from build123d import *

# Parameters (mm, degrees)
F0_W     = 88.9
F0_H     = 88.9
F0_R     = 6.35
F1_DEPTH = 12.7
F2_DEPTH = 76.2
F3_R     = 5.08


with BuildPart() as f1:
    # F0 (on Front) → F1 (new body)
    with BuildSketch(Plane.XZ):
        with Locations((-9.724989, -10.736793)):
            Rectangle(F0_W, F0_H)
        with Locations((-40.30901, -41.320814)):
            Circle(F0_R, mode=Mode.SUBTRACT)
        with Locations((20.859033, -41.320814)):
            Circle(F0_R, mode=Mode.SUBTRACT)
        with Locations((-40.30901, 19.847229)):
            Circle(F0_R, mode=Mode.SUBTRACT)
        with Locations((-9.724989, -10.736793)):
            Circle(F0_R, mode=Mode.SUBTRACT)
        with Locations((20.859033, 19.847229)):
            Circle(F0_R, mode=Mode.SUBTRACT)
    extrude(amount=-F1_DEPTH)

    # F0 (on Front) → F2 (join)
    with BuildSketch(Plane.XZ):
        with Locations((-40.30901, 19.847229)):
            Circle(F0_R)
        with Locations((20.859033, 19.847229)):
            Circle(F0_R)
        with Locations((-9.724989, -10.736793)):
            Circle(F0_R)
        with Locations((20.859033, -41.320814)):
            Circle(F0_R)
        with Locations((-40.30901, -41.320814)):
            Circle(F0_R)
    extrude(amount=-F2_DEPTH)

    # F3
    f3_edges = [f1.edges().sort_by_distance(p)[0] for p in [
        (34.725011, 6.35, 33.713207),
        (-54.174989, 6.35, 33.713207),
        (-54.174989, 6.35, -55.186793),
        (34.725011, 6.35, -55.186793),
        (14.509033, 12.7, 19.847229),
        (-46.65901, 12.7, 19.847229),
        (-16.074989, 12.7, -10.736793),
        (-46.65901, 12.7, -41.320814),
        (14.509033, 12.7, -41.320814),
    ]]
    fillet(f3_edges, radius=F3_R)


solid = f1.part
Verification items for the finished model (mm, model axes). A direction names the side the tool comes from. Round coordinates to 2 decimals unless told otherwise and drop trailing zeros. Loops run counter-clockwise (first coordinate to the right, second up) from the corner with the lowest first, then second, coordinate; pieces in that order, holes last. Notation, with made-up numbers: (9, 15) - (14, 15) arc R17 ccw to (14, 47) - close; hole circle Ø3 at (31.25, -33.5). An arc over 180 degrees is marked (long way). Answer in a Markdown table with one row per item. Add a question column.
Q1. Tool access check on faces 4 (the face through (-10, 76.2, -11)), 5 (the face through (26.916, 46.581, -39.413)). Record the directions out of +Z, -Z, +X, -X, +Y, -Y that give a thin tool (end or side, any length) a straight path to the whole face; none if there is none.
Q2. Material ranges on line 1 (Y direction, x = 25, z = -12.5); line 2 (Z direction, x = -39, y = 30); line 3 (Z direction, x = 19, y = 18), recorded low to high.
Q3. Gauge pin test, flat ends, axial feed: pin 1 (1 mm diameter, centred on y = 23, z = 20, fed in from +X); pin 2 (8 mm diameter, centred on y = 59.5, z = -34.5, fed in from -X); pin 3 (4 mm diameter, centred on x = -34.5, y = 31.5, fed in from +Z). Record the tip position at first contact, or that the pin passes through.
Q4. Section check A-A on y = 65.5. Enter the section's corners in (x, z), plus the area to 3 significant figures.
Q5. Section check C-C on x = -22.5. Enter the section's corners in (y, z).
Q6. Section check B-B on z = -24. Enter the section's corners in (x, y), plus the area to 3 significant figures.
Q7. Release check for a two-part mould opening along X. For faces 1 (the face through (21, 76.2, 20)), 2 (the face through (-41.136, 46.581, 26.143)), 3 (the face through (33.2, 6.44, 32.26)) record: pulls with the +X half, pulls with the -X half, needs draft (parallel to the pull), parting line crosses it, or undercut.
Found:
| question | item | result |
|---|---|---|
| 1 | face 4 | +Z, -Z, +X, -X, +Y |
| 1 | face 5 | +Y |
| 2 | line 1 | y = 0 to 12.7 |
| 2 | line 2 | z = -47.53 to -35.11, 13.63 to 26.06 |
| 2 | line 3 | z = -47.39 to -35.25, 13.78 to 25.92 |
| 3 | pin 1 | stops at x = 27.21 |
| 3 | pin 2 | stops at x = -46 |
| 3 | pin 3 | stops at z = 24.93 |
| 4 | outline | circle Ø12.7 at (-40.31, -41.32); circle Ø12.7 at (-40.31, 19.85); circle Ø12.7 at (-9.72, -10.74); circle Ø12.7 at (20.86, -41.32); circle Ø12.7 at (20.86, 19.85) |
| 4 | area | 633 mm² |
| 5 | outline | (0, -55.19) - (12.7, -55.19) - (12.7, 33.71) - (0, 33.71) - close |
| 6 | outline | (-54.17, 0) - (34.73, 0) - (34.73, 12.7) - (-54.17, 12.7) - close |
| 6 | area | 1,130 mm² |
| 7 | face 1 | needs draft |
| 7 | face 2 | undercut |
| 7 | face 3 | pulls with the +X half |
